Model file for the job. Use its own axes, mm. Give positions to 0.01 mm unless a question says otherwise; leave off trailing zeros. Order: outer loops, then holes, each group sorted by start corner. A loop starts at its lowest first (then second) coordinate and runs counter-clockwise, first axis right, second up. Notation, with made-up numbers: (-36, 57.25) -> (4, 57.25) arc R11 cw to (4, 62.25) -> close; hole circle Ø11 at (87, 88.5). An arc over 180 degrees is marked (long way). Answer in a Markdown table with one row per item. Add a question column.
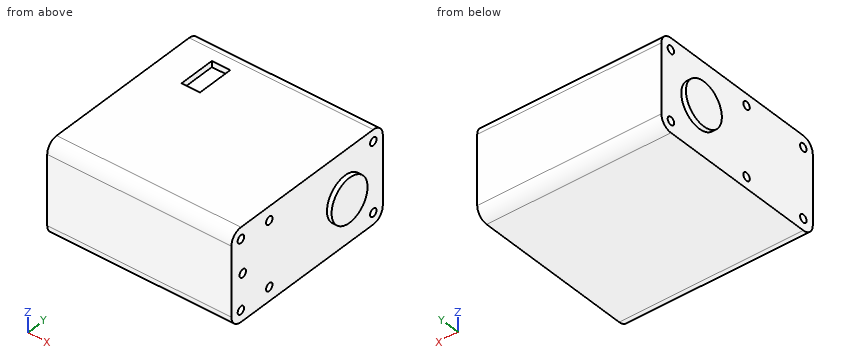
Autodesk Inventor part; units mm, degrees
ref_plane "YZ Plane" through (0, 0, 0) normal (1, 0, 0) x (0, 1, 0)
ref_plane "XZ Plane" through (0, 0, 0) normal (0, 1, 0) x (-1, 0, 0)
ref_plane "XY Plane" through (0, 0, 0) normal (0, 0, 1) x (1, 0, 0)
sketch "Base" plane through (0, 0, 0) normal (0, 0, 1) x (1, 0, 0)
  line L0 (-20, 20) -> (20, 20)
  line L1 (20, 20) -> (20, -20)
  line L2 (20, -20) -> (-20, -20)
  line L3 (-20, -20) -> (-20, 20)
  line L4 (0, 20) -> (0, -20) construction
  point P0 (0, 0)
  point P1 (0, 0)
  dimension "d0" = 40
  dimension "d1" = 40
extrude "BaseFeature" add sketch "Base" along normal mid plane 20
sketch "Axis" plane through (20, -20, 10) normal (1, 0, 0) x (0, 0, -1)
  circle A0 centre (10, 30) radius 10 construction
  line L0 (20, 40) -> (0, 40) construction
  line L1 (0, 0) -> (0, 40) construction
  circle A1 centre (10, 30) radius 4.75
  line L2 (20, 40) -> (20, 0)
  point P0 (10, 20)
  dimension "d4" = 9.5
extrude "AxisFeature" add sketch "Axis" along normal blind 1
mirror "AxisMirrorFeature" about plane through (0, 0, 0) normal (1, 0, 0) of "AxisFeature"
sketch "Sketch3" plane through (0, 0, 10) normal (0, 0, 1) x (1, 0, 0)
  line L0 (-13, 15) -> (-9, 15)
  line L1 (-9, 15) -> (-9, 7)
  line L2 (-9, 7) -> (-13, 7)
  line L3 (-13, 7) -> (-13, 15)
  line L4 (20, 20) -> (-20, 20)
  line L5 (-20, 20) -> (-20, -20)
  point P0 (0, 0)
  point P1 (-11, 15)
  dimension "d7" = 8
  dimension "d8" = 4
  dimension "d9" = 5
  dimension "d10" = 7
extrude "Extrusion3" cut sketch "Sketch3" against normal blind 1.3
fillet "Fillet1" radius 2.5 4 edges at (0, 20, 10) (0, -20, 10) (0, -20, -10) (0, 20, -10)
sketch "Sketch4" plane through (20, -17.5, 10) normal (1, 0, 0) x (0, 0, -1)
  arc A0 (2.5, 37.5) -> (0, 35) centre (2.5, 35) ccw
  arc A1 (20, 35) -> (17.5, 37.5) centre (17.5, 35) ccw
  arc A2 (0, 0) -> (2.5, -2.5) centre (2.5, 0) ccw
  arc A3 (17.5, -2.5) -> (20, 0) centre (17.5, 0) ccw
  circle A4 centre (2.5, 35) radius 0.85
  circle A5 centre (17.5, 35) radius 0.85
  circle A6 centre (2.5, 0) radius 0.85
  circle A7 centre (17.5, 0) radius 0.85
  point P0 (10, 17.5)
  dimension "d14" = 1.7
extrude "Extrusion4" cut sketch "Sketch4" against normal blind 10
mirror "Mirror2" about plane through (0, 0, 0) normal (1, 0, 0) of "Extrusion4"
sketch "Sketch6" plane through (-20, -17.5, -10) normal (-1, 0, 0) x (0, 0, 1)
  circle A0 centre (17.5, 0) radius 0.85 construction
  circle A1 centre (2.5, 0) radius 0.85 construction
  line L0 (17.5, 0) -> (2.5, 0) construction
  line L1 (2.5, 0) -> (2.5, 15) construction
  line L2 (2.5, 15) -> (17.5, 15) construction
  line L3 (17.5, 15) -> (17.5, 0) construction
  circle A2 centre (17.5, 15) radius 0.85
  circle A3 centre (2.5, 15) radius 0.85
  point P0 (10, 17.5)
  dimension "d18" = 15
extrude "Extrusion5" cut sketch "Sketch6" against normal blind 10
sketch "Sketch7" plane through (20, -17.5, 10) normal (1, 0, 0) x (0, 0, -1)
  line L0 (0, 0) -> (0, 35) construction
  line L1 (20, 35) -> (20, 0) construction
  circle A0 centre (10, 7.5) radius 10 construction
  line L2 (17.5, -2.5) -> (2.5, -2.5) construction
  circle A1 centre (10, 7.5) radius 4 construction
  line L3 (10, 17.5) -> (10, -2.5) construction
  line L4 (0, 7.5) -> (20, 7.5) construction
  line L5 (10, 11.5) -> (10, 17.5) construction
  circle A2 centre (10, 14.5) radius 0.85
  line L6 (10, 3.5) -> (10, -2.5) construction
  line L7 (20, 0) -> (20, 35)
  circle A3 centre (10, 0.5) radius 0.85
  line L8 (0, 7.5) -> (6, 7.5) construction
  line L9 (14, 7.5) -> (20, 7.5) construction
  circle A4 centre (3, 7.5) radius 0.85
  circle A5 centre (17, 7.5) radius 0.85
  circle A6 centre (2.5, 0) radius 0.85
  dimension "d21" = 8
extrude "Extrusion6" cut sketch "Sketch7" against normal blind 10 contours A3 | A4 | A5
ref_plane "Work Plane1" through (0, 0, 0) normal (1, 0, 0) x (0, 1, 0)
properties part number "FeeTechSTS3025BL"
Item 1: Pin check, flat tips, straight feed: pin 1 Ø1.9 at (y, z) = (-2.5, 7.5) entering from -X; pin 2 Ø1.4 at (y, z) = (-10, -7) entering from +X; pin 3 Ø1.5 at (y, z) = (17.5, -7.5) entering from -X. Stop position of each tip, or through.
Item 2: Wall check: line 1 (Y direction, x = -16.5, z = 7.5); line 2 (Y direction, x = 17.5, z = -7); line 3 (Z direction, x = -12, y = -2). Give the ranges that are in metal, low to high.
Item 3: Saw through at A-A on x = 18.5. List the corners of the cut face in (y, z), plus the area to 3 significant figures.
Item 4: Saw through at B-B on y = -2.5. List the corners of the cut face in (x, z).
Item 5: Saw through at C-C on x = -16.5. List the corners of the cut face in (y, z), plus the area to 3 significant figures.
Item 6: Saw through at D-D on z = 2.25. List the corners of the cut face in (x, y).
Evaluation:
| question | item | result |
|---|---|---|
| 1 | pin 1 | stops at x = -20 |
| 1 | pin 2 | stops at x = 10 |
| 1 | pin 3 | stops at x = -10 |
| 2 | line 1 | y = -20 to -18.35, -16.65 to -3.35, -1.65 to 16.65, 18.35 to 20 |
| 2 | line 2 | y = -20 to -18.19, -16.81 to -10.85, -9.15 to 16.81, 18.19 to 20 |
| 2 | line 3 | z = -10 to -8.19, -6.81 to 6.81, 8.19 to 10 |
| 3 | outline | (-20, -7.5) arc R2.5 ccw to (-17.5, -10) -> (17.5, -10) arc R2.5 ccw to (20, -7.5) -> (20, 7.5) arc R2.5 ccw to (17.5, 10) -> (-17.5, 10) arc R2.5 ccw to (-20, 7.5) -> close; hole circle Ø1.7 at (-17.5, -7.5); hole circle Ø1.7 at (-17.5, 7.5); hole circle Ø1.7 at (-17, 0); hole circle Ø1.7 at (-10, -7); hole circle Ø1.7 at (-10, 7); hole circle Ø1.7 at (17.5, -7.5); hole circle Ø1.7 at (17.5, 7.5) |
| 3 | area | 779 mm2 |
| 4 | outline | (-20, -10) -> (20, -10) -> (20, 10) -> (-20, 10) -> (-20, 8.35) -> (-10, 8.35) -> (-10, 6.65) -> (-20, 6.65) -> (-20, -6.65) -> (-10, -6.65) -> (-10, -8.35) -> (-20, -8.35) -> close |
| 5 | outline | (-20, -7.5) arc R2.5 ccw to (-17.5, -10) -> (17.5, -10) arc R2.5 ccw to (20, -7.5) -> (20, 7.5) arc R2.5 ccw to (17.5, 10) -> (-17.5, 10) arc R2.5 ccw to (-20, 7.5) -> close; hole circle Ø1.7 at (-17.5, -7.5); hole circle Ø1.7 at (-17.5, 7.5); hole circle Ø1.7 at (-2.5, -7.5); hole circle Ø1.7 at (-2.5, 7.5); hole circle Ø1.7 at (17.5, -7.5); hole circle Ø1.7 at (17.5, 7.5) |
| 5 | area | 781 mm2 |
| 6 | outline | (-21, 5.82) -> (-20, 5.82) -> (-20, -20) -> (20, -20) -> (20, 5.82) -> (21, 5.82) -> (21, 14.18) -> (20, 14.18) -> (20, 20) -> (-20, 20) -> (-20, 14.18) -> (-21, 14.18) -> close |
